Input: part model. Units: mm. Frame: model coordinates. Face numbers are marked on the shaded views. Coordinates: 2 decimals unless noted, no trailing zeros. Order: outer loops, then holes, each group sorted by start corner. A loop starts at its lowest first (then second) coordinate and runs counter-clockwise, first axis right, second up. Notation, with made-up numbers: (33.5, 9.5) -> (75.5, 9.5) arc R4 cw to (75.5, 13.5) -> close; hole circle Ø9 at (25, 15.5). An arc over 180 degrees is marked (long way). Write each question's results on one line, items separated by ' | '.
```python
from build123d import *

# Parameters (mm, degrees)
SKIZZE1_R                       = 1.5
AUFSATZ_LINEAR_AUSTRAGEN1_DEPTH = 1.5


with BuildPart() as part:
    # Skizze1 → Aufsatz-Linear austragen1 (new body, symmetric)
    with BuildSketch(Plane.XY):
        with BuildLine():
            Line((-12.5, 5.2), (-12.5, -0.5))
            Line((-12.5, -0.5), (-2.828427125, -0.5))
            ThreePointArc((-2.828427125, -0.5), (0, -4.5), (2.828427125, -0.5))
            Line((2.828427125, -0.5), (12.5, -0.5))
            Line((12.5, -0.5), (12.5, 5.2))
            Line((12.5, 5.2), (11, 5.2))
            Line((11, 5.2), (10, 3.7))
            Line((10, 3.7), (11, 3.7))
            Line((11, 3.7), (11, 1.5))
            Line((11, 1.5), (-11, 1.5))
            Line((-11, 1.5), (-11, 3.7))
            Line((-11, 3.7), (-10, 3.7))
            Line((-10, 3.7), (-11, 5.2))
            Line((-11, 5.2), (-12.5, 5.2))
        make_face()
        with Locations((0, -1.5)):
            Circle(SKIZZE1_R, mode=Mode.SUBTRACT)
    extrude(amount=AUFSATZ_LINEAR_AUSTRAGEN1_DEPTH, both=True)


solid = part.part
```
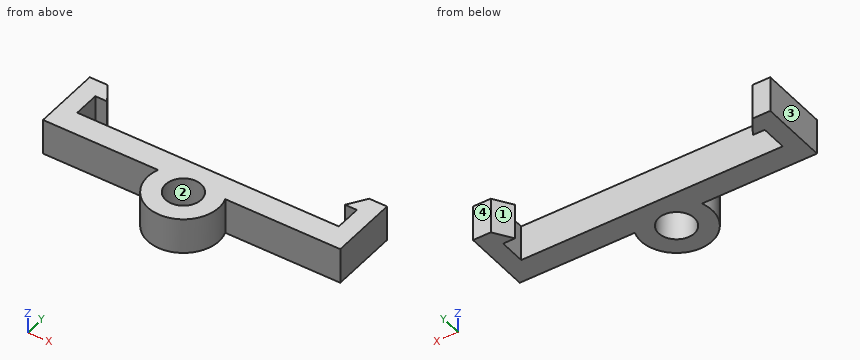
(1) Line query: line 1 along X through (y, z) = (2, 0.7); line 2 along Y through (x, z) = (7.5, 0.9); line 3 along X through (y, z) = (5, -0.8). Output: solid intervals per line, ascending. Write a range as from..to.
Return value:
line 1: -12.5..-11, 11..12.5 | line 2: -0.5..1.5 | line 3: -12.5..-10.87, 10.87..12.5
(2) Cut plane B-B, the plane y = -1.5. Return loops of the section in (x, z).
Return value:
outline: (-3, -1.5) -> (-1.5, -1.5) -> (-1.5, 1.5) -> (-3, 1.5) -> close; (1.5, -1.5) -> (3, -1.5) -> (3, 1.5) -> (1.5, 1.5) -> close
(3) Cut plane C-C, the plane z = -0.3. Return loops of the section in (x, y).
Return value:
outline: (-12.5, -0.5) -> (-2.83, -0.5) arc R3 ccw (long way) to (2.83, -0.5) -> (12.5, -0.5) -> (12.5, 5.2) -> (11, 5.2) -> (10, 3.7) -> (11, 3.7) -> (11, 1.5) -> (-11, 1.5) -> (-11, 3.7) -> (-10, 3.7) -> (-11, 5.2) -> (-12.5, 5.2) -> close; hole circle Ø3 at (0, -1.5)
(4) Pin query (flat end, axial travel): P1, Ø0.9, axis at x = 8, z = 0.5, coming from the -Y side; P2, Ø1.5, axis at x = 4, z = -0.5, coming from the +Y side; P3, Ø1, axis at x = -1.5, z = 0, coming from the -Y side. Return the tip coordinate at first contact, or that it passes through.
Return value:
P1: y = -0.5 | P2: y = 1.5 | P3: y = -4.33
(5) Cut plane D-D, the plane x = 3.25. Return loops of the section in (y, z), plus the area to 3 significant figures.
Return value:
outline: (-0.5, -1.5) -> (1.5, -1.5) -> (1.5, 1.5) -> (-0.5, 1.5) -> close | area: 6.00 mm2
(6) Mould query, pull axis X, two halves, no side actions, for the marked faces 1, 2, 3 and 4. Classes: +X half, -X half, draft (parallel to the pull), parting line (faces both ways), or undercut.
Return value:
face 1: undercut | face 2: undercut | face 3: -X half | face 4: draft
(7) Cut plane A-A, the plane x = 0. Return loops of the section in (y, z).
Return value:
outline: (-4.5, -1.5) -> (-3, -1.5) -> (-3, 1.5) -> (-4.5, 1.5) -> close; (0, -1.5) -> (1.5, -1.5) -> (1.5, 1.5) -> (0, 1.5) -> close
